from build123d import *

# Parameters (mm, degrees)
SKETCH1_R           = 13
BOSS_EXTRUDE1_DEPTH = 2.5
SKETCH3_R           = 0.4


with BuildPart() as part:
    # Sketch1 → Boss-Extrude1 (new, symmetric)
    with BuildSketch(Plane.XY):
        Circle(SKETCH1_R)
    extrude(amount=BOSS_EXTRUDE1_DEPTH, both=True)

    # Sweep1: sweep along a path in Sketch2
    with BuildLine(Plane.XY) as sweep1_path:
        Line((-2.5, 0), (-2.5, -35))
    # Sketch3 → Sweep1 (sweep)
    with BuildSketch(Plane(origin=(0, 0, 0), x_dir=(1, 0, 0), z_dir=(0, 1, 0))):
        with Locations((-2.489602721, 0)):
            Circle(SKETCH3_R)
    sweep1 = sweep(path=sweep1_path.line)

    # Mirror1: Sweep1 across plane
    add(sweep1.mirror(Plane(origin=(0, 0, 0), x_dir=(0, 0, 1), z_dir=(1, 0, 0))))


solid = part.part
Here's how the part is built. I have some questions about the finished solid (model axes, mm). Coordinates: 2 decimals unless noted, no trailing zeros. Loops run counter-clockwise (first coordinate to the right, second up) from the corner with the lowest first, then second, coordinate; pieces in that order, holes last. Notation, with made-up numbers: (-11.75, -23) -> (19.25, -23) arc R27 cw to (19.25, -7) -> close; hole circle Ø10 at (3.5, 48.25). An arc over 180 degrees is marked (long way). Use one line per item in the form item = value. Start each with the question number.
(1) Will these pins go through, and if not, where does the flat tip stop? pin 1 (10 mm diameter, centred on x = 1.5, y = -25.5, fed in from -Z); pin 2 (6 mm diameter, centred on x = -5, y = -24.5, fed in from +Z).
(2) If we section it at A-A (y = -30.5): Please give me the cut outline in (x, z).
(3) Please list where these lines run through material, in increasing order: line 1 along Y through (x, z) = (-11, -1.15); line 2 along Y through (x, z) = (8.75, -0.55); line 3 along X through (y, z) = (-8, -0.5).
(4) If we section it at D-D (y = 8): Please give me the cut outline in (x, z), then the cut area to 3 significant figures.
(5) If we section it at B-B (z = 1.45): Please give me the cut outline in (x, y), then the cut area to 3 significant figures.
(6) If we section it at C-C (x = 0): Please give me the cut outline in (y, z).
Verdict:
q1.pin_1 = -0.4
q1.pin_2 = 0.4
q2.outline = circle Ø0.8 at (-2.49, 0); circle Ø0.8 at (2.49, 0)
q3.line_1 = -6.93 to 6.93
q3.line_2 = -9.61 to 9.61
q3.line_3 = -10.25 to 10.25
q4.outline = (-10.25, -2.5) -> (10.25, -2.5) -> (10.25, 2.5) -> (-10.25, 2.5) -> close
q4.area = 102 mm²
q5.outline = circle Ø26 at (0, 0)
q5.area = 531 mm²
q6.outline = (-13, -2.5) -> (13, -2.5) -> (13, 2.5) -> (-13, 2.5) -> close
